For this review, take the finished solid that the model builds, in its own axes (mm). A direction names the side the tool comes from. Coordinates: 2 decimals unless noted, no trailing zeros. Loops run counter-clockwise (first coordinate to the right, second up) from the corner with the lowest first, then second, coordinate; pieces in that order, holes last. Notation, with made-up numbers: M -16.75,83.25 L 0.25,83.25 A22 cw 0.25,113.25 Z; hole C -22,-24.5 d2. An arc over 180 degrees is marked long. Put each result on its own line as item: value.
```python
from build123d import *

# Parameters (mm, degrees)
SKETCH1_W                       = 165.1
SKETCH1_H                       = 142.875
BOSS_EXTRUDE1_DEPTH             = 12.7
BOSS_EXTRUDE2_DEPTH             = 12.7
CUT_EXTRUDE1_REACH              = 116.135
BOSS_EXTRUDE3_DEPTH             = 12.7
F_21_0_159_DIAMETER_HOLE2_D     = 4.0386
F_21_0_159_DIAMETER_HOLE2_DEPTH = 22.225
F_21_0_159_DIAMETER_HOLE2_TIP   = 1.213317848
F_21_0_159_DIAMETER_HOLE3_D     = 4.0386
F_21_0_159_DIAMETER_HOLE3_DEPTH = 22.225
F_21_0_159_DIAMETER_HOLE3_TIP   = 1.213317848
CUT_EXTRUDE2_DEPTH              = 12.7
SKETCH21_R                      = 5.08
SKETCH21_R_2                    = 4.7752
SKETCH21_R_3                    = 11.075399998
SKETCH21_R_4                    = 3.1877
CUT_EXTRUDE10_DEPTH             = 6.35
F_8_CLEARANCE_HOLE1_D           = 4.4958
F_8_CLEARANCE_HOLE1_DEPTH       = 19.05
F_8_CLEARANCE_HOLE1_TIP         = 1.350674586
M3_CLEARANCE_HOLE1_D            = 3.4
M3_CLEARANCE_HOLE1_DEPTH        = 19.05
M3_CLEARANCE_HOLE1_TIP          = 1.021463052
SKETCH28_R                      = 11.075399998
CUT_EXTRUDE11_DEPTH             = 12.7
SKETCH29_W                      = 9.525
SKETCH29_H                      = 12.7
CUT_EXTRUDE12_DEPTH             = 115.134515622
FILLET1_R                       = 3.175
F_5_0_2055_DIAMETER_HOLE1_D     = 5.2197


with BuildPart() as part:
    # Sketch1 → Boss-Extrude1 (new body)
    with BuildSketch(Plane.XY):
        Rectangle(SKETCH1_W, SKETCH1_H)
    extrude(amount=BOSS_EXTRUDE1_DEPTH)

    # Sketch2 → Boss-Extrude2 (add)
    with BuildSketch(Plane.XY.offset(12.7)):
        Polygon((-11.1125, 71.4375), (11.1125, 71.4375), (11.1125, 75.2475), (10.664629469, 77.7875), (-10.664629469, 77.7875), (-11.1125, 75.2475), align=None)
    extrude(amount=-BOSS_EXTRUDE2_DEPTH)

    # Sketch4 → Cut-Extrude1 (cut, up to next)
    with BuildSketch(Plane.XY.offset(12.7), mode=Mode.PRIVATE) as cut_extrude1_sk1:
        with BuildLine():
            Line((-17.7165, 71.4375), (-11.1125, 71.4375))
            ThreePointArc((-11.1125, 71.4375), (-14.4145, 68.1355), (-17.7165, 71.4375))
        make_face()
    cut_extrude1_tool1 = extrude(cut_extrude1_sk1.sketch, amount=-CUT_EXTRUDE1_REACH, mode=Mode.PRIVATE) & part.part
    # Sketch4 → Cut-Extrude1 (cut, up to next)
    with BuildSketch(Plane.XY.offset(12.7), mode=Mode.PRIVATE) as cut_extrude1_sk2:
        with BuildLine():
            Line((11.1125, 71.4375), (17.7165, 71.4375))
            ThreePointArc((17.7165, 71.4375), (14.4145, 68.1355), (11.1125, 71.4375))
        make_face()
    cut_extrude1_tool2 = extrude(cut_extrude1_sk2.sketch, amount=-CUT_EXTRUDE1_REACH, mode=Mode.PRIVATE) & part.part
    add(cut_extrude1_tool1.solids().sort_by_distance((-14.4145, 70.036088, 12.7))[0], mode=Mode.SUBTRACT)
    add(cut_extrude1_tool2.solids().sort_by_distance((14.4145, 70.036088, 12.7))[0], mode=Mode.SUBTRACT)

    # Sketch5 → Boss-Extrude3 (add)
    with BuildSketch(Plane.XY.offset(12.7)):
        Polygon((63.5, -71.4375), (41.275, -71.4375), (41.275, -75.2475), (41.722870531, -77.7875), (63.052129469, -77.7875), (63.5, -75.2475), align=None)
    boss_extrude3 = extrude(amount=-BOSS_EXTRUDE3_DEPTH)

    # #21 (0.159) Diameter Hole2
    with Locations(Plane(origin=(82.55, 0, 0), x_dir=(0, 0, -1), z_dir=(1, 0, 0))):
        with Locations((-6.35, 4.7625)):
            Hole(F_21_0_159_DIAMETER_HOLE2_D / 2, depth=F_21_0_159_DIAMETER_HOLE2_DEPTH)
            with Locations((0, 0, -(F_21_0_159_DIAMETER_HOLE2_DEPTH + F_21_0_159_DIAMETER_HOLE2_TIP / 2))):  # 118° drill point
                Cone(0, F_21_0_159_DIAMETER_HOLE2_D / 2, F_21_0_159_DIAMETER_HOLE2_TIP, mode=Mode.SUBTRACT)

    # #21 (0.159) Diameter Hole3
    with Locations(Plane.ZY.offset(82.55)):
        with Locations((6.35, 4.7625)):
            Hole(F_21_0_159_DIAMETER_HOLE3_D / 2, depth=F_21_0_159_DIAMETER_HOLE3_DEPTH)
            with Locations((0, 0, -(F_21_0_159_DIAMETER_HOLE3_DEPTH + F_21_0_159_DIAMETER_HOLE3_TIP / 2))):  # 118° drill point
                Cone(0, F_21_0_159_DIAMETER_HOLE3_D / 2, F_21_0_159_DIAMETER_HOLE3_TIP, mode=Mode.SUBTRACT)

    # Sketch6 → Cut-Extrude2 (cut)
    with BuildSketch(Plane.XY.offset(12.7)):
        with BuildLine():
            Line((34.671, -71.4375), (41.275, -71.4375))
            ThreePointArc((41.275, -71.4375), (37.973, -68.1355), (34.671, -71.4375))
        make_face()
        with BuildLine():
            Line((63.5, -71.4375), (70.104, -71.4375))
            ThreePointArc((70.104, -71.4375), (66.802, -68.1355), (63.5, -71.4375))
        make_face()
    cut_extrude2 = extrude(amount=-CUT_EXTRUDE2_DEPTH, mode=Mode.SUBTRACT)

    # Mirror1: Boss-Extrude3, Cut-Extrude2 across plane
    add(boss_extrude3.mirror(Plane(origin=(0, 0, 0), x_dir=(0, 0, 1), z_dir=(1, 0, 0))))
    add(cut_extrude2.mirror(Plane(origin=(0, 0, 0), x_dir=(0, 0, 1), z_dir=(1, 0, 0))), mode=Mode.SUBTRACT)

    # Sketch21 → Cut-Extrude10 (cut)
    with BuildSketch(Plane.XY.offset(12.7)):
        with Locations((-53.594, -61.5315)):
            Circle(SKETCH21_R)
        with Locations((-57.15, 36.5125)):
            Circle(SKETCH21_R_2)
        with Locations((-53.594, -30.5435)):
            Circle(SKETCH21_R)
        with Locations((-22.606, -30.5435)):
            Circle(SKETCH21_R)
        with Locations((-22.606, -61.5315)):
            Circle(SKETCH21_R)
        with Locations((-38.1, -46.0375)):
            Circle(SKETCH21_R_3)
        with Locations((-3.263048163, -2.752650538)):
            Circle(SKETCH21_R_4)
        with Locations((31.573903673, -46.0375)):
            Circle(SKETCH21_R_3)
        with Locations((16.079903673, -30.5435)):
            Circle(SKETCH21_R)
        with Locations((47.067903673, -30.5435)):
            Circle(SKETCH21_R)
        with Locations((47.067903673, -61.5315)):
            Circle(SKETCH21_R)
        with Locations((16.079903673, -61.5315)):
            Circle(SKETCH21_R)
        with Locations((57.15, 36.5125)):
            Circle(SKETCH21_R_2)
    extrude(amount=-CUT_EXTRUDE10_DEPTH, mode=Mode.SUBTRACT)

    # #8 Clearance Hole1
    with Locations(Plane.XY.offset(12.7)):
        with Locations((-57.15, 36.5125), (57.15, 36.5125), (-3.263048163, -2.752650538)):
            Hole(F_8_CLEARANCE_HOLE1_D / 2, depth=F_8_CLEARANCE_HOLE1_DEPTH)
            with Locations((0, 0, -(F_8_CLEARANCE_HOLE1_DEPTH + F_8_CLEARANCE_HOLE1_TIP / 2))):  # 118° drill point
                Cone(0, F_8_CLEARANCE_HOLE1_D / 2, F_8_CLEARANCE_HOLE1_TIP, mode=Mode.SUBTRACT)

    # M3 Clearance Hole1
    with Locations(Plane.XY.offset(12.7)):
        with Locations((-53.594, -30.5435), (-22.606, -30.5435), (-22.606, -61.5315), (-53.594, -61.5315), (16.079903673, -61.5315), (16.079903673, -30.5435), (47.067903673, -30.5435), (47.067903673, -61.5315)):
            Hole(M3_CLEARANCE_HOLE1_D / 2, depth=M3_CLEARANCE_HOLE1_DEPTH)
            with Locations((0, 0, -(M3_CLEARANCE_HOLE1_DEPTH + M3_CLEARANCE_HOLE1_TIP / 2))):  # 118° drill point
                Cone(0, M3_CLEARANCE_HOLE1_D / 2, M3_CLEARANCE_HOLE1_TIP, mode=Mode.SUBTRACT)

    # Sketch28 → Cut-Extrude11 (cut)
    with BuildSketch(Plane.XY.offset(12.7)):
        with Locations((31.573903673, -46.0375)):
            Circle(SKETCH28_R)
        with Locations((-38.1, -46.0375)):
            Circle(SKETCH28_R)
    extrude(amount=-CUT_EXTRUDE11_DEPTH, mode=Mode.SUBTRACT)

    # Sketch29 → Cut-Extrude12 (cut, through all)
    with BuildSketch(Plane.XY.offset(12.7)):
        with Locations((-77.7875, -65.0875)):
            Rectangle(SKETCH29_W, SKETCH29_H)
        with Locations((77.7875, -65.0875)):
            Rectangle(SKETCH29_W, SKETCH29_H)
    extrude(amount=-CUT_EXTRUDE12_DEPTH, mode=Mode.SUBTRACT)

    # Fillet1
    fillet1_edges = [part.edges().sort_by_distance(p)[0] for p in [
        (-73.025, -58.7375, 6.35),
        (73.025, -58.7375, 6.35),
    ]]
    fillet(fillet1_edges, radius=FILLET1_R)

    # #5 (0.2055) Diameter Hole1 (through all)
    with Locations(Plane(origin=(0, 0, 0), x_dir=(-1, 0, 0), z_dir=(0, 0, -1))):
        with Locations((-73.025, 48.26), (73.025, 48.26), (73.025, -1.740000076), (-73.025, -1.740000076)):
            Hole(F_5_0_2055_DIAMETER_HOLE1_D / 2)


solid = part.part
```
(1) Draft analysis for pull direction X (two halves, no side actions). For faces 6 (the flat face through (-82.55, 5, 9)), 7 (the cylindrical face through (-71.282, 6.465, 5.264)), 8 (the cylindrical face through (-55.49, 38.03, 3.13)), state which applies: +X half, -X half, draft (parallel to the pull), parting line (faces both ways), or undercut.
Determined:
face 6: -X half
face 7: draft
face 8: undercut
(2) Tool access review of faces 1 (the flat face through (52, -77.788, 6)), 2 (the flat face through (73.025, -67, 6)), 3 (the flat face through (11.112, 73, 6)), 4 (the flat face through (47, -64, 6.35)), 5 (the cylindrical face through (-38.046, -68.136, 6.439)): name each direction out of +Z, -Z, +X, -X, +Y, -Y from which nothing blocks a thin tool from reaching the whole face with its end or side.
Determined:
face 1: +Z, -Z, +X, -X, -Y
face 2: +Z, -Z, +X, -Y
face 3: +Z, -Z, +X, +Y
face 4: +Z
face 5: +Z, -Z, -Y
(3) Add section A-A (y = 48.26). Write out the cut boundary in (x, z).
Determined:
outline: M -82.55,0 L -75.63,0 L -75.63,12.7 L -82.55,12.7 Z; M -70.42,0 L 70.42,0 L 70.42,12.7 L -70.42,12.7 Z; M 75.63,0 L 82.55,0 L 82.55,12.7 L 75.63,12.7 Z
(4) Wall thickness on line 1 along X through (y, z) = (48, 2); line 2 along X through (y, z) = (37.5, 6.25); line 3 along Y through (x, z) = (45, 9): over which ranges is each line inside the solid? List them lowest first. Write a range as [from, to].
Determined:
line 1: x = [-82.55, -75.62], [-70.43, 70.43], [75.62, 82.55]
line 2: x = [-82.55, -59.17], [-55.13, 55.13], [59.17, 82.55]
line 3: y = [-77.79, -66.17], [-56.89, -35.18], [-25.9, 71.44]
(5) Add section C-C (x = 24.5). Write out the cut boundary in (y, z), plus the area to 3 significant figures.
Determined:
outline: M -71.44,0 L -54.56,0 L -54.56,12.7 L -71.44,12.7 Z; M -37.52,0 L 71.44,0 L 71.44,12.7 L -37.52,12.7 Z
area: 1,600 mm^2
(6) Add section B-B (x = -36.5). Write out the cut boundary in (y, z), plus the area to 3 significant figures.
Determined:
outline: M -68.48,0 L -57,0 L -57,12.7 L -68.48,12.7 Z; M -35.08,0 L 71.44,0 L 71.44,12.7 L -35.08,12.7 Z
area: 1,500 mm^2
(7) For pin 1 (2 mm diameter, centred on x = 59.5, y = 35.5, fed in from +Z); pin 2 (2 mm diameter, centred on x = 9.5, z = 6.5, fed in from -Y); pin 3 (1.5 mm diameter, centred on x = 64.5, z = 3.5, fed in from +Y), all flat-tipped, find the tip position at first contact; note any pin that passes through.
Determined:
pin 1: stops at z = 6.35
pin 2: stops at y = -71.44
pin 3: stops at y = 71.44
